from build123d import *

# Parameters (mm, degrees)
BASE_FLANGE1_DEPTH  = 83
SKETCH2_W           = 50
SKETCH2_H           = 3.1
SKETCH2_W_2         = 25
BOSS_EXTRUDE1_DEPTH = 3
SKETCH3_W           = 138
SKETCH3_H           = 3.2
SKETCH3_W_2         = 25
BOSS_EXTRUDE2_DEPTH = 3


# Sheet-metal steps are written as plain solids
with BuildPart() as part:
    # Sketch1 → Base-Flange1 (new body)
    with BuildSketch(Plane(origin=(0, 0, 0), x_dir=(1, 0, 0), z_dir=(0, 1, 0))):
        with BuildLine():
            Line((-144, 137), (-126.171572875, 154.828427125))
            ThreePointArc((-126.171572875, 154.828427125), (-124.87387948, 155.69551813), (-123.343145751, 156))
            Line((-123.343145751, 156), (123.343145751, 156))
            ThreePointArc((123.343145751, 156), (124.87387948, 155.69551813), (126.171572875, 154.828427125))
            Line((126.171572875, 154.828427125), (142.828427125, 138.171572875))
            ThreePointArc((142.828427125, 138.171572875), (143.69551813, 136.87387948), (144, 135.343145751))
            Line((144, 135.343145751), (144, -135))
            Line((144, -135), (141, -135))
            Line((141, -135), (141, 135.343145751))
            ThreePointArc((141, 135.343145751), (140.923879533, 135.725829183), (140.707106781, 136.050252532))
            Line((140.707106781, 136.050252532), (124.050252532, 152.707106781))
            ThreePointArc((124.050252532, 152.707106781), (123.725829183, 152.923879533), (123.343145751, 153))
            Line((123.343145751, 153), (-123.343145751, 153))
            ThreePointArc((-123.343145751, 153), (-123.725829183, 152.923879533), (-124.050252532, 152.707106781))
            Line((-124.050252532, 152.707106781), (-141.878679656, 134.878679656))
            Line((-141.878679656, 134.878679656), (-144, 137))
        make_face()
    extrude(amount=BASE_FLANGE1_DEPTH)

    # Sketch2 → Boss-Extrude1 (add)
    with BuildSketch(Plane(origin=(0, 0, -156), x_dir=(-1, 0, 0), z_dir=(0, 0, -1))):
        with Locations((0, -1.55)):
            Rectangle(SKETCH2_W, SKETCH2_H)
        with Locations((-87.5, -1.55)):
            Rectangle(SKETCH2_W_2, SKETCH2_H)
        with Locations((87.5, -1.55)):
            Rectangle(SKETCH2_W_2, SKETCH2_H)
    boss_extrude1 = extrude(amount=-BOSS_EXTRUDE1_DEPTH)

    # Sketch3 → Boss-Extrude2 (add)
    with BuildSketch(Plane(origin=(144, 0, 0), x_dir=(0, 0, -1), z_dir=(1, 0, 0))):
        with Locations((0, -1.6)):
            Rectangle(SKETCH3_W, SKETCH3_H)
        with Locations((106.5, -1.6)):
            Rectangle(SKETCH3_W_2, SKETCH3_H)
        with Locations((-106.5, -1.6)):
            Rectangle(SKETCH3_W_2, SKETCH3_H)
    boss_extrude2 = extrude(amount=-BOSS_EXTRUDE2_DEPTH)

    # Mirror1: Boss-Extrude1, Boss-Extrude2 across plane
    add(boss_extrude1.mirror(Plane.ZX.offset(41.5)))
    add(boss_extrude2.mirror(Plane.ZX.offset(41.5)))


solid = part.part
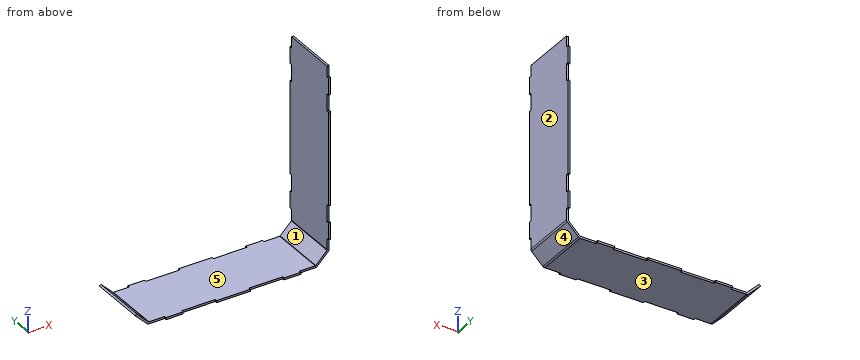
Can you work these out from the model? Positions are in its coordinate system, mm. Face numbers are marked on the shaded views. A direction names the side the tool comes from. Coordinates: 2 decimals unless noted, no trailing zeros. Write each loop counter-clockwise with the first axis right and the second up, starting at its lowest first coordinate (ties: lowest second). Pieces come first, ordered by that corner, then holes. Notation, with made-up numbers: (40, 35) -> (72, 35) arc R25 ccw to (72, 63) -> close; hole circle Ø7 at (-2, 57.25). An arc over 180 degrees is marked (long way). Answer as CSV lines item,"result".
1) Will these pins go through, and if not, where does the flat tip stop? P1, Ø10, axis at y = 57.5, z = 46, coming from the -X side; P2, Ø3.5, axis at x = 142, y = 84, coming from the -Z side; P3, Ø0.9, axis at x = 143, z = -81.5, coming from the -Y side.
Check result:
P1,"x = 141"
P2,"z = -140.44"
P3,"y = 0"
2) If I drill on line 1 (Z direction, x = -49, y = 28.5); line 2 (X direction, y = 74, z = -5); line 3 (X direction, y = 72, z = -139.5), over which ranges is the centre line in solid material (lowest first)? Write a range as from..to.
Check result:
line 1,"-156..-153"
line 2,"141..144"
line 3,"-141.5..-137.26, 137.26..141.5"
3) If we section it at A-A on y = 74: Please give me the cut outline in (x, z), then the cut area to 3 significant figures.
Check result:
outline,"(-144, -137) -> (-126.17, -154.83) arc R4 ccw to (-123.34, -156) -> (123.34, -156) arc R4 ccw to (126.17, -154.83) -> (142.83, -138.17) arc R4 ccw to (144, -135.34) -> (144, 135) -> (141, 135) -> (141, -135.34) arc R1 cw to (140.71, -136.05) -> (124.05, -152.71) arc R1 cw to (123.34, -153) -> (-123.34, -153) arc R1 cw to (-124.05, -152.71) -> (-141.88, -134.88) -> close"
area,"1,720 mm²"
4) If we section it at C-C on x = 112: Please give me the cut outline in (y, z), then the cut area to 3 significant figures.
Check result:
outline,"(0, -156) -> (83, -156) -> (83, -153) -> (0, -153) -> close"
area,"249 mm²"
5) If we section it at B-B on z = -87.5: Please give me the cut outline in (x, y).
Check result:
outline,"(141, 0) -> (144, 0) -> (144, 83) -> (141, 83) -> close"
6) If we mould it in two halves opening along X, with no side actions, what happens to the marked faces 1, 2 and 3? For each: +X half, -X half, draft (parallel to the pull), parting line (faces both ways), or undercut.
Check result:
face 1,"undercut"
face 2,"+X half"
face 3,"draft"
7) On a 3-axis mill with a long thin cutter (end or side, diameter ignored), from which of +Z, -Z, +X, -X, +Y, -Y can I reach the whole of each face in a straight line? I mean the marked faces 4 and 5. Say none if no direction works.
Check result:
face 4,"-Z, +X, +Y, -Y"
face 5,"+Z, +Y, -Y"
